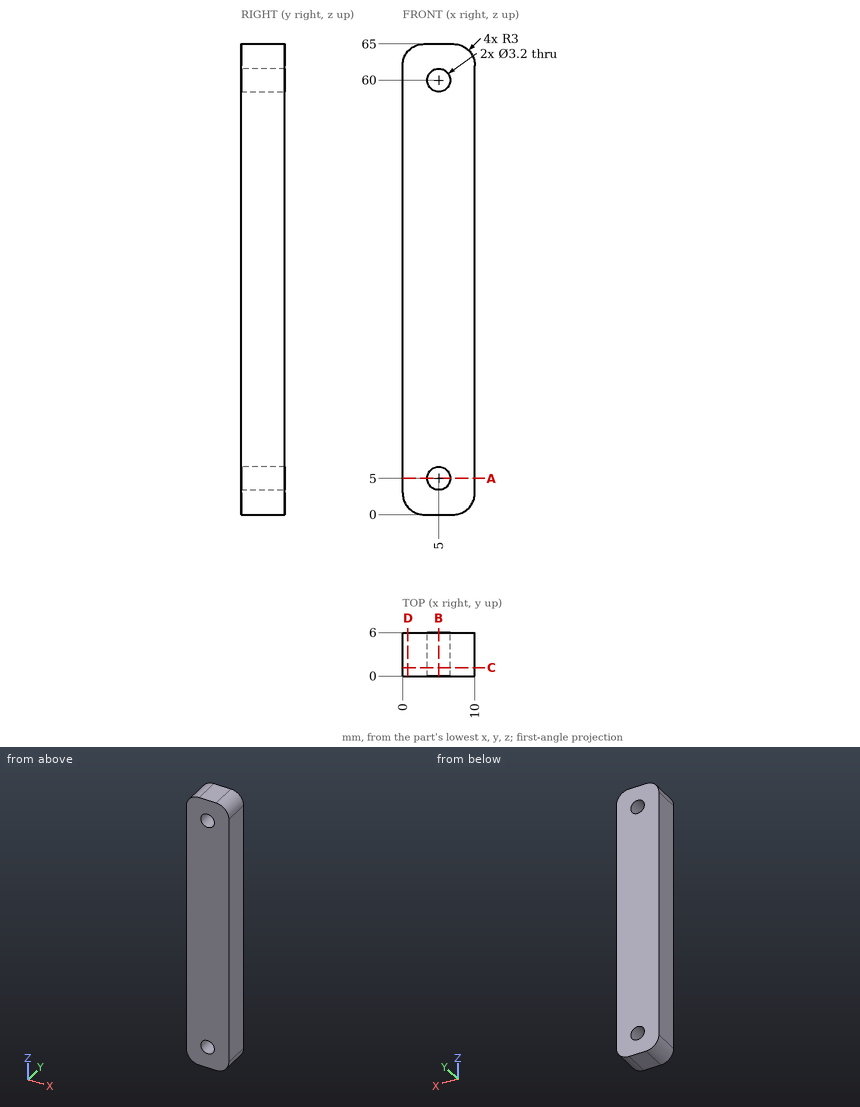
Study the drawing (mm; zero at the part's minimum x, y, z) and answer. Round coordinates to 2 decimals unless told otherwise and drop trailing zeros. Order: outer loops, then holes, each group sorted by start corner. A loop starts at its lowest first (then second) coordinate and runs counter-clockwise, first axis right, second up. Notation, with made-up numbers: M 67.5,1 L 96.5,1 A21 ccw 96.5,23 Z; hole C 46.5,30 d8. An arc over 180 degrees is marked long. One line per item, written item: value.
Q1. Find section B-B on x = 5. Write down the section's boundary in (y, z).
Derived:
outline: M 0,0 L 6,0 L 6,3.4 L 0,3.4 Z; M 0,6.6 L 6,6.6 L 6,58.4 L 0,58.4 Z; M 0,61.6 L 6,61.6 L 6,65 L 0,65 Z
Q2. Straight lines are drawn through the part: line 1 (X direction, y = 4.7, z = 5); line 2 (Z direction, x = 4.25, y = 3.1); line 3 (X direction, y = 0.7, z = 61). For each, find the intervals that lie inside material, in ascending order.
Derived:
line 1: 0 to 3.4, 6.6 to 10
line 2: 0 to 3.59, 6.41 to 58.59, 61.41 to 65
line 3: 0 to 3.75, 6.25 to 10
Q3. Flat-ended cylindrical pins translate along their axes: pin 1 (3 mm diameter, centred on x = 5, z = 60, fed in from -Y); pin 2 (1.5 mm diameter, centred on x = 9, y = 3, fed in from +Z); pin 3 (1.5 mm diameter, centred on x = 1.5, y = 1, fed in from +Z); pin 4 (1 mm diameter, centred on x = 8.5, y = 3, fed in from +Z). Find the tip coordinate at first contact, or state that the pin passes through.
Derived:
pin 1: through
pin 2: z = 64.73
pin 3: z = 64.9
pin 4: z = 64.83
Q4. Find section C-C on y = 1.15. Write down the section's boundary in (x, z), then the cut area to 3 significant figures.
Derived:
outline: M 0,3 A3 ccw 3,0 L 7,0 A3 ccw 10,3 L 10,62 A3 ccw 7,65 L 3,65 A3 ccw 0,62 Z; hole C 5,5 d3.2; hole C 5,60 d3.2
area: 626 mm²
Q5. Find section A-A on z = 5. Write down the section's boundary in (x, y).
Derived:
outline: M 0,0 L 3.4,0 L 3.4,6 L 0,6 Z; M 6.6,0 L 10,0 L 10,6 L 6.6,6 Z
Q6. Find section D-D on x = 0.75. Write down the section's boundary in (y, z), then the cut area to 3 significant figures.
Derived:
outline: M 0,1.02 L 6,1.02 L 6,63.98 L 0,63.98 Z
area: 378 mm²
